Autodesk Inventor part; units mm, degrees
ref_plane "YZ Plane" through (0, 0, 0) normal (1, 0, 0) x (0, 1, 0)
ref_plane "XZ Plane" through (0, 0, 0) normal (0, 1, 0) x (-1, 0, 0)
ref_plane "XY Plane" through (0, 0, 0) normal (0, 0, 1) x (1, 0, 0)
sketch "Sketch1" plane through (0, 0, 0) normal (0, 0, 1) x (1, 0, 0)
  line L0 (-79, -79) -> (79, -79)
  line L1 (79, -79) -> (79, 79)
  line L2 (79, 79) -> (-79, 79)
  line L3 (-79, 79) -> (-79, -79)
  line L4 (-79, 0) -> (0, 0) construction
  line L5 (0, 0) -> (0, -79) construction
  point P0 (0, -79)
  dimension "d0" = 158
  dimension "d1" = 158
extrude "Extrusion1" add sketch "Sketch1" along normal blind 9.525
sketch "Sketch2" plane through (0, 0, 9.525) normal (0, 0, 1) x (1, 0, 0)
  circle A0 centre (0, 0) radius 68 construction
  line L0 (0, 0) -> (0, -68) construction
  circle A1 centre (0, 0) radius 68 construction
  circle A2 centre (0, 0) radius 68 construction
  circle A3 centre (0, 0) radius 68 construction
  circle A4 centre (0, 0) radius 68 construction
  point P0 (64.6718, -21.0132)
  point P1 (64.6718, -21.0132)
  point P2 (39.9694, 55.0132)
  point P3 (39.9694, 55.0132)
  point P4 (-39.9694, 55.0132)
  point P5 (-39.9694, 55.0132)
  point P6 (-64.6718, -21.0132)
  point P7 (-64.6718, -21.0132)
  dimension "d4" = 136
  dimension "d7" = 360
hole "Hole1" at (0, -68, 9.525) at (64.6718, -21.0132, 9.525) at (39.9694, 55.0132, 9.525) at (-39.9694, 55.0132, 9.525) at (-64.6718, -21.0132, 9.525) direction (0, 0, -1) diameter 5 end through all
sketch "Sketch4" plane through (0, 0, 9.525) normal (0, 0, 1) x (1, 0, 0)
  line L0 (79, -79) -> (79, 79) construction
  line L1 (79, 79) -> (-79, 79) construction
  line L2 (-79, 79) -> (-79, -79) construction
  line L3 (-79, -79) -> (79, -79) construction
  line L4 (-79, 0) -> (79, 0) construction
  line L5 (0, 79) -> (0, -79) construction
  circle A0 centre (0, 0) radius 63
  dimension "d16" = 126
extrude "Extrusion2" cut sketch "Sketch4" against normal through all
sketch "Sketch5" plane through (-79, -79, 0) normal (0, -1, 0) x (1, 0, 0)
  line L0 (158, 0) -> (158, 9.525) construction
  line L1 (0, 9.525) -> (158, 9.525) construction
  line L2 (0, 0) -> (158, 0) construction
  line L3 (0, 0) -> (0, 9.525) construction
  line L4 (0, 4.7625) -> (158, 4.7625) construction
  point P0 (79, 0)
  point P1 (31.6, 4.7625)
  point P2 (126.4, 4.7625)
  point P3 (94.8, 4.7625)
  point P4 (63.2, 4.7625)
  dimension "d19" = 31.6
  dimension "d20" = 31.6
  dimension "d21" = 31.6
  dimension "d22" = 31.6
  dimension "d23" = 31.6
hole "Hole2" at (-47.4, -79, 4.7625) at (47.4, -79, 4.7625) at (15.8, -79, 4.7625) at (-15.8, -79, 4.7625) direction (0, 1, 0) diameter 4.978 depth 19.05 tip angle 118
properties part number "face_part"
Work out the finished part from the listing and answer in its coordinate system (mm). A direction names the side the tool comes from. Round coordinates to 2 decimals unless told otherwise and drop trailing zeros. Write each loop counter-clockwise with the first axis right and the second up, starting at its lowest first coordinate (ties: lowest second). Pieces come first, ordered by that corner, then holes. Notation, with made-up numbers: (-26, -37.5) - (-22, -37.5) arc R29 ccw to (-22, -4.5) - close; hole circle Ø8 at (38, -20.5). An arc over 180 degrees is marked (long way). Return JSON: item names as keys, results as strings. Group by question number.
Q1. For faces 4 (the flat face through (-36, 54, 9.525)), 5 (the cylindrical face through (-49.868, -69.342, 5.087)), determine the directions among +Z, -Z, +X, -X, +Y, -Y from which every point of the face is accessible in a straight line to the end or side of a thin tool.
Q2. The part is cut by section A-A on y = -68. Write down the section's boundary in (x, z) (1 decimal).
Q3. Each of these flat-tipped pins is pushed along its axis until it touches: pin 1 Ø4 at (x, y) = (-39.97, 55.01) entering from -Z; pin 2 Ø4.5 at (x, z) = (15.8, 4.76) entering from -Y; pin 3 Ø3 at (x, z) = (-47.4, 4.76) entering from -Y. Where does it stop, or does it pass through?
Q4. The part is cut by section D-D on x = -55.5. Write down the section's boundary in (y, z) (3 decimals), then the cut area to 3 significant figures.
Q5. The mould has two halves that part along Y. Classify faces 1 (the cylindrical face through (66.89, -22.17, 4.7)), 2 (the cylindrical face through (18.23, -69.51, 5.3)), 3 (the conical face through (-47.822, -58.714, 4.856)): released by +Y, released by -Y, zero draft, split by the parting line, or undercut.
Q6. The part is cut by section B-B on x = 0. Write down the section's boundary in (y, z) (3 decimals).
Q7. Find the intervals of material crossed by L1, parallel to Y at x = 0, z = 4.5; L2, parallel to Y at x = 2, z = 1.5; L3, parallel to X at y = -38.5, z = 1.5, in increasing order.
Q8. The part is cut by section C-C on y = 0. Write down the section's boundary in (x, z) (3 decimals), then the cut area to 3 significant figures.
Solved:
{
 "1": {"face 4": "+Z, +X, -X, +Y, -Y", "face 5": "-Y"},
 "2": {"outline": "(-79, 0) - (-2.5, 0) - (-2.5, 9.5) - (-79, 9.5) - close; (2.5, 0) - (79, 0) - (79, 9.5) - (2.5, 9.5) - close; hole circle Ø5 at (-47.4, 4.8); hole circle Ø5 at (-15.8, 4.8); hole circle Ø5 at (15.8, 4.8); hole circle Ø5 at (47.4, 4.8)"},
 "3": {"pin 1": "through", "pin 2": "y = 60.36", "pin 3": "y = -59.36"},
 "4": {"outline": "(-79, 0) - (-29.812, 0) - (-29.812, 9.525) - (-79, 9.525) - close; (29.812, 0) - (79, 0) - (79, 9.525) - (29.812, 9.525) - close", "area": "937 mm²"},
 "5": {"face 1": "undercut", "face 2": "zero draft", "face 3": "released by -Y"},
 "6": {"outline": "(-79, 0) - (-70.5, 0) - (-70.5, 9.525) - (-79, 9.525) - close; (-65.5, 0) - (-63, 0) - (-63, 9.525) - (-65.5, 9.525) - close; (63, 0) - (79, 0) - (79, 9.525) - (63, 9.525) - close"},
 "7": {"L1": "-79 to -70.5, -65.5 to -63, 63 to 79", "L2": "-79 to -69.5, -66.5 to -62.97, 62.97 to 79", "L3": "-79 to -49.87, 49.87 to 79"},
 "8": {"outline": "(-79, 0) - (-63, 0) - (-63, 9.525) - (-79, 9.525) - close; (63, 0) - (79, 0) - (79, 9.525) - (63, 9.525) - close", "area": "305 mm²"}
}
